```python
from build123d import *

# Parameters (mm, degrees)
BOSS_EXTRUDE1_DEPTH           = 12.75
BOSS_EXTRUDE1_DEPTH_BACK      = 12.75
SKETCH1_W                     = 165
SKETCH1_H                     = 100
SKETCH5_W                     = 6
SKETCH5_H                     = 13
CUT_EXTRUDE3_DEPTH            = 19.25
SKETCH6_R                     = 10.25
CUT_EXTRUDE4_DEPTH            = 105.029133509
SKETCH11_R                    = 1.5
CUT_EXTRUDE6_DEPTH            = 5
SKETCH2_R                     = 6.63
SKETCH2_R_2                   = 3.525
SKETCH2_R_3                   = 1.975
CUT_EXTRUDE7_DEPTH            = 131.264394598
SKETCH3_R                     = 2.5
CUT_EXTRUDE8_DEPTH            = 5
SKETCH12_R                    = 0.985
CUT_EXTRUDE9_DEPTH            = 5
MOVE_START                    = -12.75
MOVE_FACE1_DEPTH              = 25.5
MOVE_FACE1_2_DEPTH            = 20.5
SKETCH13_W                    = 10
SKETCH13_H                    = 20
CUT_EXTRUDE10_DEPTH           = 107.491783721
CHAMFER1_SIZE                 = 2
SKETCH14_R                    = 1.5
CUT_EXTRUDE11_DEPTH           = 5
CUT_EXTRUDE12_START           = -5
SKETCH15_R                    = 1.5
CUT_EXTRUDE12_DEPTH           = 5
CUT_EXTRUDE15_START           = -25.5
SKETCH17_R                    = 1.5
CUT_EXTRUDE15_DEPTH           = 132.991783721
SKETCH18_R                    = 1.475
SKETCH18_R_2                  = 1.5
CUT_EXTRUDE16_DEPTH           = 5
SKETCH16_R                    = 1
CUT_EXTRUDE13_DEPTH           = 10
CBORE_FOR_M3_SHCS1_AT_2_COUNT = 2
CBORE_FOR_M3_SHCS1_AT_2_PITCH = 43.77
CBORE_FOR_M3_SHCS1_AT_3_COUNT = 2
CBORE_FOR_M3_SHCS1_AT_3_PITCH = 80.030074972
CBORE_FOR_M3_SHCS1_AT_4_COUNT = 2
CBORE_FOR_M3_SHCS1_AT_4_PITCH = 67


# Read off the part's stored shape, not the designer's step: Move Face1
with BuildPart() as part:
    # Sketch1 → Boss-Extrude1 (new, two sides: drawn at the far end of the back side and taken through both)
    with BuildSketch(Plane(origin=(0, 0, 0), x_dir=(1, 0, 0), z_dir=(0, 1, 0)).offset(-BOSS_EXTRUDE1_DEPTH_BACK)):
        Rectangle(SKETCH1_W, SKETCH1_H)
    extrude(amount=BOSS_EXTRUDE1_DEPTH + BOSS_EXTRUDE1_DEPTH_BACK)

    # Sketch5 → Cut-Extrude3 (cut)
    with BuildSketch(Plane(origin=(82.5, 0, 0), x_dir=(0, 0, -1), z_dir=(1, 0, 0))):
        with Locations((-30, 0)):
            Rectangle(SKETCH5_W, SKETCH5_H)
        with Locations((30, 0)):
            Rectangle(SKETCH5_W, SKETCH5_H)
    extrude(amount=-CUT_EXTRUDE3_DEPTH, mode=Mode.SUBTRACT)

    # Sketch6 → Cut-Extrude4 (cut, through all)
    with BuildSketch(Plane(origin=(0, 20.916044041, 3.688062894), x_dir=(1, 0, 0), z_dir=(0, 0.984807753012208, 0.17364817766693072))):
        with Locations(Location((0, -21.249093385, 0), (0, 0, 270))):
            Circle(SKETCH6_R)
    extrude(amount=-CUT_EXTRUDE4_DEPTH, mode=Mode.SUBTRACT)

    # Sketch11 → Cut-Extrude6 (cut)
    with BuildSketch(Plane(origin=(0, 12.75, 0), x_dir=(1, 0, 0), z_dir=(0, 1, 0))):
        with Locations(Location((-28.466991411, -15.483495706, 0), (0, 0, 270))):
            Circle(SKETCH11_R)
        with Locations(Location((-54.983495706, -42, 0), (0, 0, 270))):
            Circle(SKETCH11_R)
        with Locations(Location((-54.983495706, 11.033008589, 0), (0, 0, 90))):
            Circle(SKETCH11_R)
        with Locations((-81.5, -15.483495706)):
            Circle(SKETCH11_R)
    extrude(amount=-CUT_EXTRUDE6_DEPTH, mode=Mode.SUBTRACT)

    # Sketch2 → Cut-Extrude7 (cut, through all)
    with BuildSketch(Plane.XY.offset(50)):
        with Locations((-69.75, 0)):
            Circle(SKETCH2_R)
        with Locations((69.75, 0)):
            Circle(SKETCH2_R_2)
        with Locations(Location((-75.45, -8.2, 0), (0, 0, 180))):
            Circle(SKETCH2_R_3)
        with Locations(Location((-62.05, 8.2, 0), (0, 0, 180))):
            Circle(SKETCH2_R_3)
    extrude(amount=-CUT_EXTRUDE7_DEPTH, mode=Mode.SUBTRACT)

    # Sketch3 → Cut-Extrude8 (cut)
    with BuildSketch(Plane(origin=(0, 12.75, 0), x_dir=(1, 0, 0), z_dir=(0, 1, 0))):
        with Locations(Location((-15, -4.8, 0), (0, 0, 270))):
            Circle(SKETCH3_R)
        with Locations(Location((67.72, -4.8, 0), (0, 0, 270))):
            Circle(SKETCH3_R)
        with Locations(Location((60.37, 43.46, 0), (0, 0, 270))):
            Circle(SKETCH3_R)
        with Locations(Location((-14.76, 43.46, 0), (0, 0, 270))):
            Circle(SKETCH3_R)
    extrude(amount=-CUT_EXTRUDE8_DEPTH, mode=Mode.SUBTRACT)

    # Sketch12 → Cut-Extrude9 (cut)
    with BuildSketch(Plane(origin=(0, 12.75, 0), x_dir=(1, 0, 0), z_dir=(0, 1, 0))):
        with Locations(Location((-56.672, 32.8, 0), (0, 0, 270))):
            Circle(SKETCH12_R)
        with Locations(Location((-72.039, 17.2, 0), (0, 0, 270))):
            Circle(SKETCH12_R)
    extrude(amount=-CUT_EXTRUDE9_DEPTH, mode=Mode.SUBTRACT)

    # Move Face1 outline → Move Face1 (add)
    with BuildSketch(Plane(origin=(0, 0, 0), x_dir=(1, 0, 0), z_dir=(0, 1, 0)).offset(MOVE_START)):
        with BuildLine():
            Line((-82.5, 50), (-90.5, 50))
            Line((-90.5, 50), (-90.5, -50))
            Line((-90.5, -50), (-82.5, -50))
            Line((-82.5, -50), (-82.5, -16.601529694))
            ThreePointArc((-82.5, -16.601529694), (-83, -15.483495706), (-82.5, -14.365461717))
            Line((-82.5, -14.365461717), (-82.5, 50))
        make_face()
    extrude(amount=MOVE_FACE1_DEPTH)

    # Move Face1 2 outline → Move Face1 2 (add)
    with BuildSketch(Plane(origin=(0, 0, 0), x_dir=(1, 0, 0), z_dir=(0, 1, 0)).offset(MOVE_START)):
        with BuildLine():
            Line((-82.5, -16.601529694), (-82.5, -14.365461717))
            ThreePointArc((-82.5, -14.365461717), (-83, -15.483495706), (-82.5, -16.601529694))
        make_face()
    extrude(amount=MOVE_FACE1_2_DEPTH)

    # Sketch13 → Cut-Extrude10 (cut, through all)
    with BuildSketch(Plane(origin=(0, 12.75, 0), x_dir=(1, 0, 0), z_dir=(0, 1, 0))):
        with Locations((45.5, -30)):
            Rectangle(SKETCH13_W, SKETCH13_H)
    extrude(amount=-CUT_EXTRUDE10_DEPTH, mode=Mode.SUBTRACT)

    # Chamfer1
    chamfer1_edges = [part.edges().sort_by_distance(p)[0] for p in [
        (40.5, 0, 40),
        (40.5, 0, 20),
        (50.5, 0, 20),
        (50.5, 0, 40),
    ]]
    chamfer(chamfer1_edges, length=CHAMFER1_SIZE)

    # Sketch14 → Cut-Extrude11 (cut)
    with BuildSketch(Plane(origin=(82.5, 0, 0), x_dir=(0, 0, -1), z_dir=(1, 0, 0))):
        with Locations((0, 2.75)):
            Circle(SKETCH14_R)
    extrude(amount=-CUT_EXTRUDE11_DEPTH, mode=Mode.SUBTRACT)

    # Sketch15 → Cut-Extrude12 (cut)
    with BuildSketch(Plane.ZY.offset(90.5).offset(CUT_EXTRUDE12_START)):
        with Locations(Location((0, 2.75, 0), (0, 0, 180))):
            Circle(SKETCH15_R)
    extrude(amount=CUT_EXTRUDE12_DEPTH, mode=Mode.SUBTRACT)

    # Sketch17 → Cut-Extrude15 (cut, through all)
    with BuildSketch(Plane(origin=(0, 12.75, 0), x_dir=(1, 0, 0), z_dir=(0, 1, 0)).offset(CUT_EXTRUDE15_START)):
        with Locations(Location((33.5, -1.940063906, 0), (0, 0, 90))):
            Circle(SKETCH17_R)
        with Locations(Location((33.5, -45.710063906, 0), (0, 0, 90))):
            Circle(SKETCH17_R)
        with Locations(Location((-33.5, -45.710063906, 0), (0, 0, 90))):
            Circle(SKETCH17_R)
        with Locations(Location((-33.5, -1.940063906, 0), (0, 0, 90))):
            Circle(SKETCH17_R)
    extrude(amount=CUT_EXTRUDE15_DEPTH, mode=Mode.SUBTRACT)

    # Sketch18 → Cut-Extrude16 (cut)
    with BuildSketch(Plane.XZ.offset(12.75)):
        with Locations(Location((31, -38.46, 0), (0, 0, 270))):
            Circle(SKETCH18_R)
        with Locations(Location((72, -21, 0), (0, 0, 270))):
            Circle(SKETCH18_R_2)
        with Locations(Location((72, -41, 0), (0, 0, 90))):
            Circle(SKETCH18_R_2)
        with Locations(Location((-10, -21, 0), (0, 0, 90))):
            Circle(SKETCH18_R_2)
        with Locations(Location((-10, -41, 0), (0, 0, 270))):
            Circle(SKETCH18_R_2)
    extrude(amount=-CUT_EXTRUDE16_DEPTH, mode=Mode.SUBTRACT)

    # Sketch16 → Cut-Extrude13 (cut)
    with BuildSketch(Plane(origin=(82.5, 0, 0), x_dir=(0, 0, -1), z_dir=(1, 0, 0))):
        with Locations((42.508182421, -6.590003662)):
            Circle(SKETCH16_R)
        with Locations((42.508182421, 1.409996338)):
            Circle(SKETCH16_R)
    extrude(amount=-CUT_EXTRUDE13_DEPTH, mode=Mode.SUBTRACT)

    # Sketch22 → CBORE for M3 SHCS1 (revolve, cut)
    with BuildSketch(Plane(origin=(33.5, 12.75, 1.940063906), x_dir=(0, 0, 1), z_dir=(1, 0, 0))):
        Polygon((0, 0), (0, 25.5), (1.8, 25.5), (1.8, 20), (3.25, 20), (3.25, 0.025), (3.275, 0), align=None)
    cbore_for_m3_shcs1 = revolve(axis=Axis((33.5, 19.1, 1.940063906), (0, -1, 0)), mode=Mode.SUBTRACT)

    # CBORE for M3 SHCS1 at 2: CBORE for M3 SHCS1 ×2
    with Locations(*[(0, 0, i * CBORE_FOR_M3_SHCS1_AT_2_PITCH) for i in range(1, CBORE_FOR_M3_SHCS1_AT_2_COUNT)]):
        add(cbore_for_m3_shcs1, mode=Mode.SUBTRACT)

    # CBORE for M3 SHCS1 at 3: CBORE for M3 SHCS1 ×2
    with Locations(*[Vector(-0.8371852709567797, 0, 0.5469193926832577) * (i * CBORE_FOR_M3_SHCS1_AT_3_PITCH) for i in range(1, CBORE_FOR_M3_SHCS1_AT_3_COUNT)]):
        add(cbore_for_m3_shcs1, mode=Mode.SUBTRACT)

    # CBORE for M3 SHCS1 at 4: CBORE for M3 SHCS1 ×2
    with Locations(*[(-i * CBORE_FOR_M3_SHCS1_AT_4_PITCH, 0, 0) for i in range(1, CBORE_FOR_M3_SHCS1_AT_4_COUNT)]):
        add(cbore_for_m3_shcs1, mode=Mode.SUBTRACT)


solid = part.part
```
Design review of the part built by this model. Coordinates are the model's own, in mm. A direction names the side the tool comes from. Give positions to 0.01 mm unless a question says otherwise; leave off trailing zeros. Order: outer loops, then holes, each group sorted by start corner. A loop starts at its lowest first (then second) coordinate and runs counter-clockwise, first axis right, second up. Notation, with made-up numbers: (29.25, 73) -> (41.25, 73) arc R22 cw to (41.25, 83) -> close; hole circle Ø10 at (78.25, -22). An arc over 180 degrees is marked (long way). Write item = value, one per line. Start each with the question number.
(1) We need section A-A on x = -66. Write out the cut boundary in (y, z), plus the area to 3 significant figures.
(2) For faces 4 (the face through (-15, 7.75, 5)), 5 (the face through (63.25, 0, -30)), 6 (the face through (-60.077, 8.113, 0.7)), 7 (the face through (40.5, 0, 30)), list the 3-axis set-ups (+Z, -Z, +X, -X, +Y, -Y) from which the entire face can be reached by the end or side of a thin tool; tool diameter is ignored.
(3) For pin 1 (2 mm diameter, centred on x = -33.5, z = 45.71, fed in from +Y); pin 2 (1.8 mm diameter, centred on x = -28.47, z = 15.48, fed in from +Y), all flat-tipped, find the tip position at first contact; note any pin that passes through.
(4) Mouldability with a two-part tool opening along Y and no side actions: class faces 1 (the face through (75, 0, -33)), 2 (the face through (62.48, 10.28, -42.12)), 3 (the face through (35, -7.25, 44)) as +Y half, -Y half, draft (parallel to the pull), parting line (faces both ways), or undercut.
(5) To check wall thickness, follow line 1 along X through (y, z) = (-11.4, -41); line 2 along X through (y, z) = (-8.25, 29); line 3 along Z through (x, y) = (32, 5). State the ranges of each line that lie inside material, in increasing order.
Numbers:
q1.outline = (-12.75, -50) -> (-5.47, -50) -> (-5.47, 50) -> (-12.75, 50) -> close; (5.47, -50) -> (12.75, -50) -> (12.75, 50) -> (5.47, 50) -> close
q1.area = 1,460 mm^2
q2.face_4 = +Y
q2.face_5 = +X
q2.face_6 = +Z, -Z
q2.face_7 = +Y, -Y
q3.pin_1 = through
q3.pin_2 = 7.75
q4.face_1 = undercut
q4.face_2 = draft
q4.face_3 = +Y half
q5.line_1 = -90.5 to -11.5, -8.5 to 70.5, 73.5 to 82.5
q5.line_2 = -90.5 to -77.42, -73.48 to -5.35, 5.35 to 40.5, 50.5 to 82.5
q5.line_3 = -50 to -0.94, 4.82 to 42.83, 48.59 to 50
